Can you work these out from the model? Positions are in its coordinate system, mm. Round coordinates to 2 decimals unless told otherwise and drop trailing zeros. Write each loop counter-clockwise with the first axis right and the second up, starting at its lowest first coordinate (ties: lowest second). Pieces come first, ordered by that corner, then holes.
Q1. If we section it at A-A (x = -137.75): Please give me the cut outline in (y, z) (3 decimals), plus the area to 3 significant figures.
Q2. If we section it at B-B (y = 0.95): Please give me the cut outline in (x, z) (3 decimals).
Q3. I'm going to push flat-ended pins straight in: pin 1 Ø4 at (x, z) = (-137.5, 15) entering from -Y; pin 2 Ø1.5 at (x, y) = (-140, 1) entering from -Z; pin 3 Ø0.9 at (x, y) = (-138.5, 2) entering from +Z (3 decimals); pin 4 Ø0.9 at (y, z) = (1.5, -25.5) entering from +X. Where does each tip first touch, or does it pass through?
Q4. If we section it at C-C (x = -140.25): Please give me the cut outline in (y, z) (3 decimals), plus the area to 3 significant figures.
Q5. If we section it at D-D (z = -0.5): Please give me the cut outline in (x, y).
Q6. Please list where these lines run through material, in increasing order: line 1 along Z through (x, y) = (-137, 1.2) (3 decimals); line 2 along Z through (x, y) = (-129.75, 0.5) (3 decimals); line 3 along X through (y, z) = (0.65, 23).
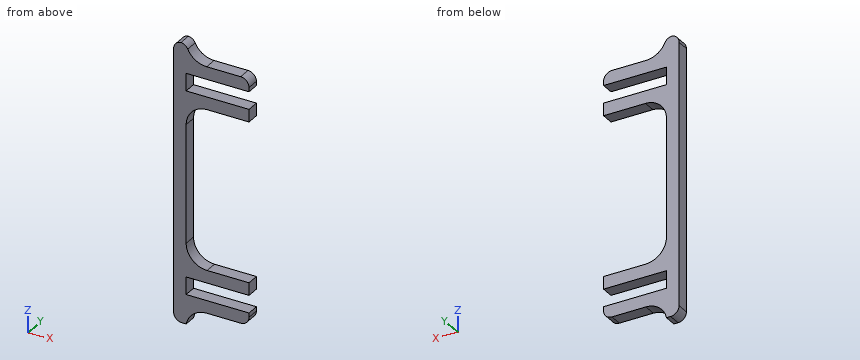
from build123d import *

# Parameters (mm, degrees)
BOSS_EXTRUDE1_DEPTH = 3
FILLET1_R           = 5
FILLET2_R           = 2


with BuildPart() as part:
    # Sketch2 → Boss-Extrude1 (new body)
    with BuildSketch(Plane(origin=(0, 0, 0), x_dir=(1, 0, 0), z_dir=(0, 1, 0))):
        Polygon((-128.893875, -24.675), (-143.893875, -24.675), (-143.893875, -20.5), (-128.893875, -20.5), (-128.893875, -17.5), (-143.893875, -17.5), (-143.893875, 20.69), (-128.893875, 20.69), (-128.893875, 23.69), (-143.893875, 23.69), (-143.893875, 27.865), (-128.893875, 27.865), (-128.893875, 30.865), (-143.893875, 30.865), (-143.893875, 34.865), (-146.893875, 34.865), (-146.893875, -31.675), (-143.893875, -31.675), (-143.893875, -27.675), (-128.893875, -27.675), align=None)
    extrude(amount=BOSS_EXTRUDE1_DEPTH)

    # Fillet1
    # the kernel refuses this fillet: 5 mm, written as the material it adds along each edge
    with BuildSketch(Plane(origin=(-143.893875, 0, 27.675), x_dir=(1.4566126083077746e-12, 0, 1.0), z_dir=(0, 1, 0))) as fillet1_piece_1:
        with BuildLine():
            CenterArc((5, 4.898979486), FILLET1_R, 180, 78.463040967)
            Line((0, 4.898979486), (-0.1, 4.898979486))
            Line((-0.1, 4.898979486), (-0.1, 0))
            Line((-0.1, 0), (0, -0.1))
            ThreePointArc((0, -0.1), (2, -0.1), (3.98, -0.09797959))
            Line((3.98, -0.09797959), (4, 0))
        make_face()
    extrude(amount=3)
    with BuildSketch(Plane(origin=(-143.893875, 0, -30.865), x_dir=(1, 0, 0), z_dir=(0, 1, 0))) as fillet1_piece_2:
        with BuildLine():
            CenterArc((4.898979486, 5), FILLET1_R, 191.536959033, 78.463040967)
            Line((0, 4), (-0.09797959, 3.98))
            ThreePointArc((-0.09797959, 3.98), (-0.1, 2), (-0.1, 0))
            Line((-0.1, 0), (0, -0.1))
            Line((0, -0.1), (4.898979486, -0.1))
            Line((4.898979486, -0.1), (4.898979486, 0))
        make_face()
    extrude(amount=3)
    with BuildSketch(Plane(origin=(-143.893875, 0, -20.69), x_dir=(0, 0, 1), z_dir=(0, 1, 0)), Plane(origin=(-143.893875, 0, 17.5), x_dir=(1, 0, 0), z_dir=(0, 1, 0))) as fillet1_piece_3:
        with BuildLine():
            CenterArc((FILLET1_R, FILLET1_R), FILLET1_R, 180, 90)
            Line((0, FILLET1_R), (-FILLET1_R * 0.02, FILLET1_R))
            Line((-FILLET1_R * 0.02, FILLET1_R), (-FILLET1_R * 0.02, -FILLET1_R * 0.02))
            Line((-FILLET1_R * 0.02, -FILLET1_R * 0.02), (FILLET1_R, -FILLET1_R * 0.02))
            Line((FILLET1_R, -FILLET1_R * 0.02), (FILLET1_R, 0))
        make_face()
    extrude(amount=3)

    # Fillet2
    # the kernel refuses this fillet: 2 mm, written as the material it takes off along each edge
    with BuildSketch(Plane(origin=(-128.893875, -5, 27.675), x_dir=(-1, 0, 0), z_dir=(0, 1, 0)), Plane(origin=(-128.893875, -5, -30.865), x_dir=(0, 0, 1), z_dir=(0, 1, 0)), Plane(origin=(-146.893875, -5, -34.865), x_dir=(1, 0, 0), z_dir=(0, 1, 0)), Plane(origin=(-146.893875, -5, 31.675), x_dir=(0, 0, -1), z_dir=(0, 1, 0))) as fillet2_piece_1:
        with BuildLine():
            CenterArc((FILLET2_R, -FILLET2_R), FILLET2_R, 90, 90)
            Line((0, -FILLET2_R), (0, 0))
            Line((0, 0), (FILLET2_R, 0))
        make_face()
    extrude(amount=13, mode=Mode.SUBTRACT)
    with BuildSketch(Plane(origin=(-143.893875, -3.563939587, 31.675), x_dir=(-1, 0, 0), z_dir=(0, 1, 0))) as fillet2_piece_2:
        with BuildLine():
            CenterArc((1.425575835, -2), FILLET2_R, 90, 64.623066475)
            ThreePointArc((-0.381439971, -1.142857143), (-0.156170388, -0.582959844), (0, 0))
            Line((0, 0), (1.425575835, 0))
        make_face()
    extrude(amount=10.127879174, mode=Mode.SUBTRACT)


solid = part.part
A:
1. outline: (0, -30.865) - (3, -30.865) - (3, -27.865) - (0, -27.865) - close; (0, -23.69) - (3, -23.69) - (3, -20.69) - (0, -20.69) - close; (0, 17.5) - (3, 17.5) - (3, 20.5) - (0, 20.5) - close; (0, 24.675) - (3, 24.675) - (3, 27.675) - (0, 27.675) - close
1. area: 36.0 mm2
2. outline: (-146.894, -32.865) arc R2 ccw to (-144.894, -34.865) - (-143.894, -34.865) arc R5 cw to (-138.995, -30.865) - (-130.894, -30.865) arc R2 ccw to (-128.894, -28.865) - (-128.894, -27.865) - (-143.894, -27.865) - (-143.894, -23.69) - (-128.894, -23.69) - (-128.894, -20.69) - (-138.894, -20.69) arc R5 cw to (-143.894, -15.69) - (-143.894, 12.5) arc R5 cw to (-138.894, 17.5) - (-128.894, 17.5) - (-128.894, 20.5) - (-143.894, 20.5) - (-143.894, 24.675) - (-128.894, 24.675) - (-128.894, 25.675) arc R2 ccw to (-130.894, 27.675) - (-138.995, 27.675) arc R5 cw to (-143.512, 30.532) arc R2 ccw to (-145.107, 31.664) arc R2 ccw to (-146.894, 29.675) - close
3. pin 1: passes through
3. pin 2: stops at z = -31.18
3. pin 3: stops at z = 27.675
3. pin 4: stops at x = -143.89
4. outline: (0, -31.025) - (3, -31.025) - (3, -27.865) - (0, -27.865) - close; (0, -23.69) - (3, -23.69) - (3, -20.503) - (0, -20.503) - close; (0, 17.313) - (3, 17.313) - (3, 20.5) - (0, 20.5) - close; (0, 24.675) - (3, 24.675) - (3, 27.835) - (0, 27.835) - close
4. area: 38.1 mm2
5. outline: (-146.89, 0) - (-143.89, 0) - (-143.89, 3) - (-146.89, 3) - close
6. line 1: z = -30.865 to -27.865, -23.69 to -20.69, 17.5 to 20.5, 24.675 to 27.675
6. line 2: z = -30.506 to -27.865, -23.69 to -20.69, 17.5 to 20.5, 24.675 to 27.316
6. line 3: x = -146.89 to -143.89
